from build123d import *

# Parameters (mm, degrees)
SKETCH1_R           = 5
BOSS_EXTRUDE1_DEPTH = 20
SKETCH2_R           = 1.35
CUT_EXTRUDE1_DEPTH  = 6
SKETCH12_R          = 1.35
CUT_EXTRUDE2_DEPTH  = 10


with BuildPart() as part:
    # Sketch1 → Boss-Extrude1 (new body)
    with BuildSketch(Plane(origin=(0, 0, 0), x_dir=(1, 0, 0), z_dir=(0, 1, 0))):
        Circle(SKETCH1_R)
    extrude(amount=BOSS_EXTRUDE1_DEPTH)

    # Sketch2 → Cut-Extrude1 (cut)
    with BuildSketch(Plane(origin=(0, 20, 0), x_dir=(1, 0, 0), z_dir=(0, 1, 0))):
        Circle(SKETCH2_R)
    extrude(amount=-CUT_EXTRUDE1_DEPTH, mode=Mode.SUBTRACT)

    # Sketch12 → Cut-Extrude2 (cut)
    with BuildSketch(Plane.XZ):
        Circle(SKETCH12_R)
    extrude(amount=-CUT_EXTRUDE2_DEPTH, mode=Mode.SUBTRACT)


solid = part.part
Source: CAD feature listing. Evaluate the final solid. Frame: model axes, mm. A direction names the side the tool comes from. Coordinates: 2 decimals unless noted, no trailing zeros. Loops run counter-clockwise (first coordinate to the right, second up) from the corner with the lowest first, then second, coordinate; pieces in that order, holes last. Notation, with made-up numbers: (42.25, -26.5) - (65.25, -26.5) arc R20 cw to (65.25, -12.5) - close; hole circle Ø1 at (-30.5, 60.5). An arc over 180 degrees is marked (long way). One line per item, written item: value. Start each with the question number.
1. Mould query, pull axis X, two halves, no side actions, for faces 1 (the cylindrical face through (-0.29, 17.04, 1.32)), 2 (the cylindrical face through (-1.08, 9.86, 4.88)), 3 (the flat face through (-1.2, 0, 1)). Classes: pulls with the +X half, pulls with the -X half, needs draft (parallel to the pull), parting line crosses it, or undercut.
2. Contact query for flat-ended pins moving along their axis: P1, Ø3, axis at y = 11.5, z = 3.5, coming from the -X side; P2, Ø1.5, axis at x = 1, y = 3.5, coming from the -Z side; P3, Ø5, axis at y = 17.5, z = 3, coming from the -X side. Output: stop coordinate, or through.
3. Set-up query: faces 4 (the flat face through (0, 14, 0)), 5 (the cylindrical face through (-0.29, 4.93, -1.32)), 6 (the flat face through (-1.2, 20, 1)). Return all of +Z, -Z, +X, -X, +Y, -Y with unobstructed straight access to the full face (end or side cutting, diameter ignored); none if empty.
4. Section D-D (x = -3). Return the cut outline in (y, z), and give its area (3 significant figures).
5. Section B-B (x = 0). Return the cut outline in (y, z).
6. Section C-C (y = 2.75). Return the cut outline in (x, z).
7. Ray query, L1, parallel to X at y = 15.4, z = 0; L2, parallel to Y at x = 0.5, z = -0.75. Return the intervals inside material, ascending.
8. Section A-A (z = 0). Return the cut outline in (x, y), and give its area (3 significant figures).
Verdict:
1. face 1: undercut
1. face 2: parting line crosses it
1. face 3: needs draft
2. P1: stops at x = -4.58
2. P2: stops at z = -4.99
2. P3: stops at x = -4.97
3. face 4: +Y
3. face 5: -Y
3. face 6: +Z, -Z, +X, -X, +Y
4. outline: (0, -4) - (20, -4) - (20, 4) - (0, 4) - close
4. area: 160 mm2
5. outline: (0, -5) - (20, -5) - (20, -1.35) - (14, -1.35) - (14, 1.35) - (20, 1.35) - (20, 5) - (0, 5) - (0, 1.35) - (10, 1.35) - (10, -1.35) - (0, -1.35) - close
6. outline: circle Ø10 at (0, 0); hole circle Ø2.7 at (0, 0)
7. L1: x = -5 to -1.35, 1.35 to 5
7. L2: y = 10 to 14
8. outline: (-5, 0) - (-1.35, 0) - (-1.35, 10) - (1.35, 10) - (1.35, 0) - (5, 0) - (5, 20) - (1.35, 20) - (1.35, 14) - (-1.35, 14) - (-1.35, 20) - (-5, 20) - close
8. area: 157 mm2
